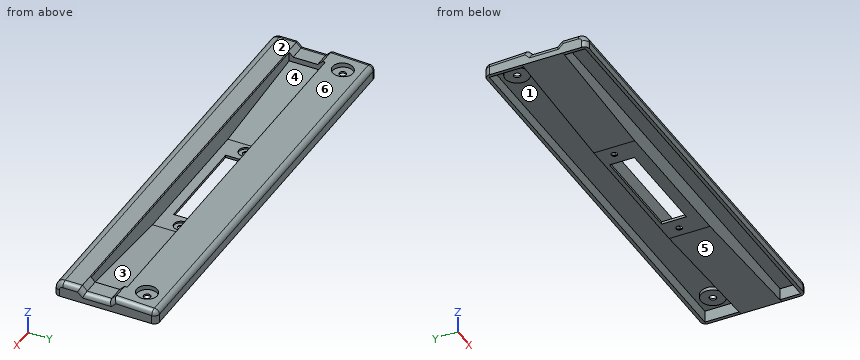
from build123d import *

# Parameters (mm, degrees)
F0_W         = 250
F0_H         = 60
F1_DEPTH     = 9
F2_W         = 86
F2_H         = 4
F3_DEPTH     = 16
F4_DEPTH     = 7.9
F5_W         = 59.5
F5_H         = 14.5
F6_DEPTH     = 13.001
F7_R         = 1.7543464605
F8_DEPTH     = 13.001
F9_W         = 246
F9_H         = 20.1
F9_H_2       = 12
F10_DEPTH    = 7
F11_R        = 1.9
F12_DEPTH    = 2.001
F14_R        = 7
F15_DEPTH    = 2
F13_R        = 6
F16_DEPTH    = 3
F17_R        = 2
F18_DEPTH    = 25
F19_W        = 86
F19_H        = 21
F20_DEPTH    = 11.5
F22_DEPTH    = 21
F24_DEPTH    = 250.001
F25_R        = 3
F26_T1_DEPTH = 250
F26_T4_ANGLE = 90
F26_T6_ANGLE = 90
F27_R        = 4
F28_DEPTH    = 1


# Not quite as in the source:
# - a fillet or chamfer that OpenCascade refuses, or shapes differently, is made with other operations: its cross-section is extruded or revolved along the edge and cut away or added


with BuildPart() as f1:
    # F0 (on Top) → F1 (new body)
    with BuildSketch(Plane.XY):
        Rectangle(F0_W, F0_H)
    extrude(amount=F1_DEPTH)

    # F2 (on Front) → F3 (join)
    with BuildSketch(Plane.XZ):
        Polygon((-43, 0), (-125, 0), (-43, -4), align=None)
        with Locations((0, -2)):
            Rectangle(F2_W, F2_H)
        Polygon((125, 0), (43, 0), (43, -4), align=None)
    extrude(amount=F3_DEPTH)

    # F2 (on Front) → F4 (join)
    with BuildSketch(Plane.XZ):
        Polygon((-43, 0), (-125, 0), (-43, -4), align=None)
        with Locations((0, -2)):
            Rectangle(F2_W, F2_H)
        Polygon((125, 0), (43, 0), (43, -4), align=None)
    extrude(amount=-F4_DEPTH)

    # F5 (on face) → F6 (cut, through all)
    with BuildSketch(Plane.XY.offset(9)):
        with Locations((0, -1.75)):
            Rectangle(F5_W, F5_H)
    extrude(amount=-F6_DEPTH, mode=Mode.SUBTRACT)

    # F7 (on face) → F8 (cut, through all)
    with BuildSketch(Plane(origin=(0, 0, -4), x_dir=(1, 0, 0), z_dir=(0, 0, -1))):
        with Locations((-37, 1)):
            Circle(F7_R)
        with Locations((37, 1)):
            Circle(F7_R)
    extrude(amount=-F8_DEPTH, mode=Mode.SUBTRACT)

    # F9 (on face) → F10 (cut)
    with BuildSketch(Plane(origin=(0, 0, 0), x_dir=(1, 0, 0), z_dir=(0, 0, -1))):
        with Locations((0, -17.95)):
            Rectangle(F9_W, F9_H)
        with Locations((0, 22)):
            Rectangle(F9_W, F9_H_2)
    extrude(amount=-F10_DEPTH, mode=Mode.SUBTRACT)

    # F11 (on face) → F12 (cut, through all)
    with BuildSketch(Plane(origin=(0, 0, 7), x_dir=(1, 0, 0), z_dir=(0, 0, -1))):
        with Locations((-111.75, -17.5)):
            Circle(F11_R)
        with Locations((111.75, -17.5)):
            Circle(F11_R)
    extrude(amount=-F12_DEPTH, mode=Mode.SUBTRACT)

    # F14 (on face) → F15 (join)
    with BuildSketch(Plane(origin=(0, 0, 7), x_dir=(1, 0, 0), z_dir=(0, 0, -1))):
        with Locations((-111.75, -17.5)):
            Circle(F14_R)
        with Locations((111.75, -17.5)):
            Circle(F14_R)
    extrude(amount=F15_DEPTH)

    # F13 (on face) → F16 (cut)
    with BuildSketch(Plane.XY.offset(9)):
        with Locations((-111.75, 17.5)):
            Circle(F13_R)
        with Locations((111.75, 17.5)):
            Circle(F13_R)
    extrude(amount=-F16_DEPTH, mode=Mode.SUBTRACT)

    # F17 (on face) → F18 (cut)
    with BuildSketch(Plane.XY.offset(6)):
        with Locations((111.75, 17.5)):
            Circle(F17_R)
        with Locations((-111.75, 17.5)):
            Circle(F17_R)
    extrude(amount=-F18_DEPTH, mode=Mode.SUBTRACT)

    # F19 (on face) → F20 (cut)
    with BuildSketch(Plane.XY.offset(9)):
        with Locations((0, -4)):
            Rectangle(F19_W, F19_H)
    extrude(amount=-F20_DEPTH, mode=Mode.SUBTRACT)

    # F21 (on face) → F22 (cut)
    with BuildSketch(Plane(origin=(0, -14.5, 0), x_dir=(-1, 0, 0), z_dir=(0, 1, 0))):
        Polygon((113, 9), (43, 9), (43, -2.5), (113, 3), align=None)
        Polygon((-43, -2.5), (-43, 9), (-113, 9), (-113, 3), align=None)
    extrude(amount=F22_DEPTH, mode=Mode.SUBTRACT)

    # F23 (on face) → F24 (cut, through all)
    with BuildSketch(Plane.YZ.offset(125)):
        Polygon((2.1715728753, 6.1715728753), (5, 9), (-15, 9), (-12.1715728753, 6.1715728753), align=None)
        Polygon((5, 9), (30, 8), (30, 9), align=None)
    extrude(amount=-F24_DEPTH, mode=Mode.SUBTRACT)

    # F25
    f25_edges = [f1.edges().sort_by_distance(p)[0] for p in [
        (125, -22.5, 9),
        (0, 30, 8),
        (-125, -22.5, 9),
        (125, -13.585786, 7.585786),
        (125, -5, 6.171573),
        (125, 3.585786, 7.585786),
        (-125, 3.585786, 7.585786),
        (-125, -5, 6.171573),
        (-125, -13.585786, 7.585786),
        (-125, 30, 4),
        (-125, -30, 4.5),
        (125, -30, 4.5),
        (125, 30, 4),
        (125, 17.5, 8.5),
        (-125, 17.5, 8.5),
    ]]
    fillet(f25_edges, radius=F25_R)

    # F26: fillet of radius 5 on 1 edges, made by hand

    # F26_s2 → F26_t1 (cut)
    with BuildSketch(Plane.YZ.offset(-125)):
        with BuildLine():
            ThreePointArc((-30, 4), (-28.5355339059, 7.5355339059), (-25, 9))
            Line((-25, 9), (-30, 9))
            Line((-30, 9), (-30, 4))
        make_face()
    extrude(amount=F26_T1_DEPTH, mode=Mode.SUBTRACT)

    # F26_s3 → F26_t4 (revolve, cut)
    with BuildSketch(Plane.XY.offset(4)):
        with BuildLine():
            ThreePointArc((-125, -27), (-124.1213203436, -29.1213203436), (-122, -30))
            Line((-122, -30), (-125, -30))
            Line((-125, -30), (-125, -27))
        make_face()
    revolve(axis=Axis((-125, -25, 4), (-1, 0, 0)), revolution_arc=F26_T4_ANGLE, mode=Mode.SUBTRACT)

    # F26_s5 → F26_t6 (revolve, cut)
    with BuildSketch(Plane.XZ.offset(25)):
        with BuildLine():
            ThreePointArc((125, 6), (124.1213203436, 8.1213203436), (122, 9))
            Line((122, 9), (125, 9))
            Line((125, 9), (125, 6))
        make_face()
    revolve(axis=Axis((125, -25, 4), (1, 0, 0)), revolution_arc=F26_T6_ANGLE, mode=Mode.SUBTRACT)

    # F27 (on face) → F28 (cut)
    with BuildSketch(Plane.XY.offset(-2.5)):
        with Locations((37, -1)):
            Circle(F27_R)
        with Locations((-37, -1)):
            Circle(F27_R)
    extrude(amount=-F28_DEPTH, mode=Mode.SUBTRACT)


solid = f1.part
CAD build for the part. Positions are in the model's coordinates, mm. Face numbers are marked on the shaded views. A direction names the side the tool comes from. Coordinates: 2 decimals unless noted, no trailing zeros. Write each loop counter-clockwise with the first axis right and the second up, starting at its lowest first coordinate (ties: lowest second). Pieces come first, ordered by that corner, then holes. Notation, with made-up numbers: M -14,-29.5 L 43,-29.5 A17 cw 43,-3.5 Z; hole C 7,47.5 d5. An arc over 180 degrees is marked long. Answer as a JSON object with one key per item and string values. Group by question number.
1) Pin check, flat tips, straight feed: pin 1 Ø4 at (x, y) = (-36.5, -1) entering from +Z; pin 2 Ø8 at (x, y) = (9.5, 23.5) entering from -Z; pin 3 Ø1.8 at (y, z) = (-4, 6) entering from +X; pin 4 Ø2.5 at (x, y) = (111.75, 17.5) entering from +Z. Stop position of each tip, or through.
2) Tool access for the marked faces 1, 2 and 3: list every direction of +Z, -Z, +X, -X, +Y, -Y with a clear straight run to the whole face (end or side of a thin tool).
3) Wall check: line 1 (Y direction, x = 111.75, z = 5.6); line 2 (Y direction, x = -16.5, z = 1); line 3 (Y direction, x = 37.5, z = -2). Give the ranges that are in metal, low to high. Write a range as from..to.
4) Mould opens along Y. For the marked faces 4, 5 and 6 say: +Y half, -Y half, draft (parallel to the pull), parting line (faces both ways), or undercut.
5) Saw through at A-A (x = -9). Write the cut outline in (y, z), plus the area to 3 significant figures.
6) Saw through at B-B (x = -94). Write the cut outline in (y, z).
Values follow:
{
 "1": {"pin 1": "stops at z = -3.5", "pin 2": "stops at z = 7", "pin 3": "stops at x = 124.3", "pin 4": "passes through"},
 "2": {"face 1": "-Z", "face 2": "+Z, +X, -X, +Y, -Y", "face 3": "+Z"},
 "3": {"line 1": "y = -29.74..-28, -16..-14.5, 6.5..7.9, 10.5..15.5, 19.5..24.5, 28..29.96", "line 2": "y = -30..-28, -16..-14.5, 6.5..7.9, 28..30", "line 3": "y = -16..-14.5, 6.5..7.9"},
 "4": {"face 4": "undercut", "face 5": "draft", "face 6": "+Y half"},
 "5": {"outline": "M -30,0 L -28,0 L -28,7 L -16,7 L -16,-4 L -9,-4 L -9,-2.5 L -14.5,-2.5 L -14.5,8.5 L -15,9 L -25,9 A5 ccw -30,4 Z; M 5.5,-4 L 7.9,-4 L 7.9,7 L 28,7 L 28,0 L 30,0 L 30,5.12 A3 ccw 27.12,8.12 L 6.5,8.94 L 6.5,-2.5 L 5.5,-2.5 Z", "area": "128 mm2"},
 "6": {"outline": "M -30,0 L -28,0 L -28,7 L -16,7 L -16,-1.51 L 7.9,-1.51 L 7.9,7 L 28,7 L 28,0 L 30,0 L 30,5.12 A3 ccw 27.12,8.12 L 6.5,8.94 L 6.5,1.51 L -14.5,1.51 L -14.5,8.5 L -15,9 L -25,9 A5 ccw -30,4 Z"}
}
